Part print with two shaded views. Sizes in mm from the minimum x, y, z corner. Round coordinates to 2 decimals unless told otherwise and drop trailing zeros. Loops run counter-clockwise (first coordinate to the right, second up) from the corner with the lowest first, then second, coordinate; pieces in that order, holes last. Notation, with made-up numbers: M 11.25,51 L 24.25,51 A4 ccw 24.25,58 Z; hole C 14,23.25 d10. An arc over 180 degrees is marked long. Answer as CSV lines item,"result". Start each with the question number.
Item 1: Wall check: line 1 (X direction, y = 39, z = 1); line 2 (Y direction, x = 67.5, z = 8.5). Give the ranges that are in metal, low to high.
Item 2: Band-saw the part on B-B (x = 261). Give the cut face in (y, z).
Item 3: Band-saw the part on A-A (z = 14.5). Give the cut face in (x, y), and give its area (3 significant figures).
Item 4: Drop flat-ended pins along their axis: pin 1 Ø3 at (y, z) = (33.5, 14.5) entering from -X; pin 2 Ø6 at (x, z) = (195.5, 6.5) entering from +Y; pin 3 Ø10 at (x, z) = (82.5, 11) entering from -Y. Give the stop position or say it passes through.
Item 5: Band-saw the part on C-C (y = 115). Give the cut face in (x, z).
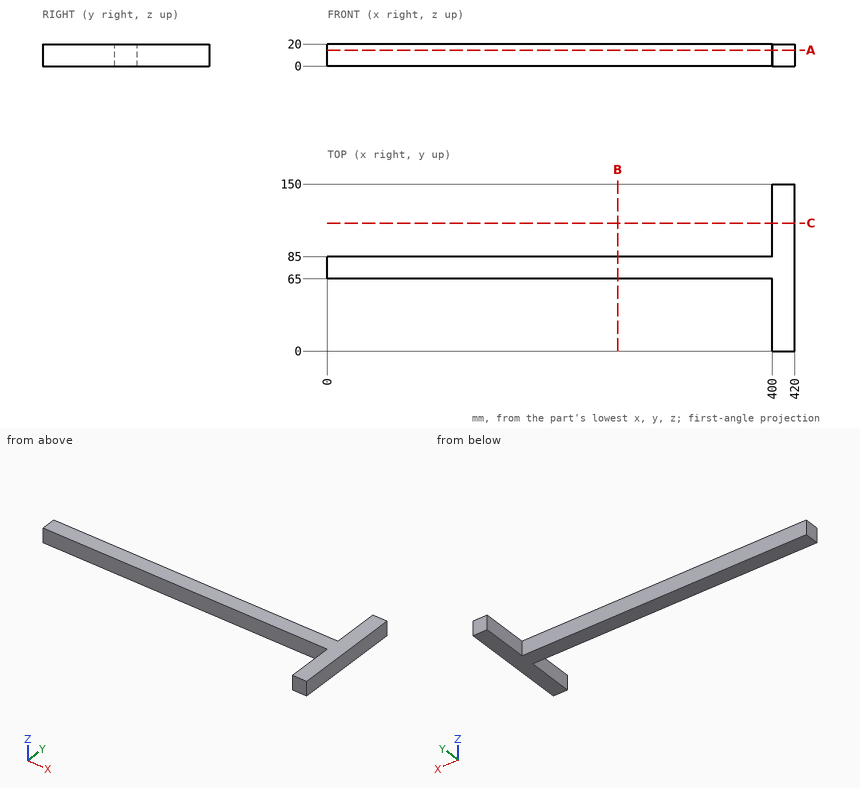
Answer block:
1,line 1,"x = 400 to 420"
1,line 2,"y = 65 to 85"
2,outline,"M 65,0 L 85,0 L 85,20 L 65,20 Z"
3,outline,"M 0,65 L 400,65 L 400,0 L 420,0 L 420,150 L 400,150 L 400,85 L 0,85 Z"
3,area,"11,000 mm^2"
4,pin 1,"stops at x = 400"
4,pin 2,"stops at y = 85"
4,pin 3,"stops at y = 65"
5,outline,"M 400,0 L 420,0 L 420,20 L 400,20 Z"
